The model under review builds one solid part; all positions refer to its coordinate system, in mm. A direction names the side the tool comes from. Round coordinates to 2 decimals unless told otherwise and drop trailing zeros. Loops run counter-clockwise (first coordinate to the right, second up) from the corner with the lowest first, then second, coordinate; pieces in that order, holes last. Notation, with made-up numbers: M 85,-11 L 143,-11 A8 ccw 143,1 Z; hole C 84.25,85 d7. An arc over 180 degrees is marked long. One line per question, with ' | ' between items.
from build123d import *

# Parameters (mm, degrees)
BOSS_EXTRUDE1_DEPTH = 9.525
BOSS_EXTRUDE2_START = -3.175
BOSS_EXTRUDE2_DEPTH = 3.175
FILLET1_R           = 9.525
SKETCH2_R           = 4.7625
SKETCH2_R_2         = 3.175
CUT_EXTRUDE1_DEPTH  = 71.245753875
SKETCH2_4_R         = 3.175
CUT_EXTRUDE2_DEPTH  = 71.245753961
CUT_EXTRUDE4_START  = -12.7
SKETCH2_6_R         = 4.7625
SKETCH2_6_R_2       = 3.175
CUT_EXTRUDE4_DEPTH  = 58.545753961


with BuildPart() as part:
    # Sketch1 → Boss-Extrude1 (new body)
    with BuildSketch(Plane.ZY.offset(50.8)):
        with BuildLine():
            ThreePointArc((12.636340451, 186.18), (-12.7, 187.45), (12.636340451, 188.72))
            Line((12.636340451, 188.72), (26.9875, 188.72))
            Line((26.9875, 188.72), (26.9875, 193.8))
            Line((26.9875, 193.8), (16.267034341, 193.8))
            ThreePointArc((16.267034341, 193.8), (-17.4625, 187.45), (16.267034341, 181.1))
            Line((16.267034341, 181.1), (26.9875, 181.1))
            Line((26.9875, 181.1), (26.9875, 186.18))
            Line((26.9875, 186.18), (12.636340451, 186.18))
        make_face()
    extrude(amount=BOSS_EXTRUDE1_DEPTH)

    # Sketch1<4> → Boss-Extrude2 (add)
    with BuildSketch(Plane.ZY.offset(50.8).offset(BOSS_EXTRUDE2_START)):
        with BuildLine():
            Line((17.416256953, 186.18), (14.256444382, 186.18))
            ThreePointArc((14.256444382, 186.18), (-14.3129, 187.45), (14.256444382, 188.72))
            Line((14.256444382, 188.72), (17.416256953, 188.72))
            ThreePointArc((17.416256953, 188.72), (17.032105803, 191.303086834), (16.267034341, 193.8))
            ThreePointArc((16.267034341, 193.8), (-17.4625, 187.45), (16.267034341, 181.1))
            ThreePointArc((16.267034341, 181.1), (17.032105803, 183.596913166), (17.416256953, 186.18))
        make_face()
        with BuildLine():
            ThreePointArc((16.267034341, 193.8), (17.032105803, 191.303086834), (17.416256953, 188.72))
            Line((17.416256953, 188.72), (26.9875, 188.72))
            Line((26.9875, 188.72), (26.9875, 193.8))
            Line((26.9875, 193.8), (16.267034341, 193.8))
        make_face()
        with BuildLine():
            Line((26.9875, 186.18), (17.416256953, 186.18))
            ThreePointArc((17.416256953, 186.18), (17.032105803, 183.596913166), (16.267034341, 181.1))
            Line((16.267034341, 181.1), (26.9875, 181.1))
            Line((26.9875, 181.1), (26.9875, 186.18))
        make_face()
    extrude(amount=BOSS_EXTRUDE2_DEPTH)

    # Fillet1
    fillet1_edges = [part.edges().sort_by_distance(p)[0] for p in [
        (-53.975, 181.1, 16.267034341),
        (-53.975, 193.8, 16.267034341),
    ]]
    fillet(fillet1_edges, radius=FILLET1_R)

    # Sketch2 → Cut-Extrude1 (cut, through all)
    # profile 1 of 2: a face of its own
    with BuildSketch(Plane(origin=(0, 193.8, 0), x_dir=(1, 0, 0), z_dir=(0, 1, 0))):
        with Locations((-53.975, -21.62726717)):
            Circle(SKETCH2_R)
        with Locations((-53.975, -21.62726717)):
            Circle(SKETCH2_R_2, mode=Mode.SUBTRACT)
    # profile 2 of 2: a face of its own
    with BuildSketch(Plane(origin=(0, 193.8, 0), x_dir=(1, 0, 0), z_dir=(0, 1, 0))):
        with Locations((-53.975, -21.62726717)):
            Circle(SKETCH2_R_2)
    extrude(amount=CUT_EXTRUDE1_DEPTH, mode=Mode.SUBTRACT)

    # Sketch2<4> → Cut-Extrude2 (cut, through all)
    with BuildSketch(Plane(origin=(0, 193.8, 0), x_dir=(1, 0, 0), z_dir=(0, 1, 0))):
        with Locations(Location((-53.975, -21.62726717, 0), (0, 0, 270))):
            Circle(SKETCH2_4_R)
    extrude(amount=-CUT_EXTRUDE2_DEPTH, mode=Mode.SUBTRACT)

    # Sketch2<6> → Cut-Extrude4 (cut, through all)
    # profile 1 of 3: a face of its own
    with BuildSketch(Plane(origin=(0, 193.8, 0), x_dir=(1, 0, 0), z_dir=(0, 1, 0)).offset(CUT_EXTRUDE4_START)):
        Polygon((-60.325, -21.513289799), (-60.325, -21.741244542), (-57.296072999, -26.9875), (-50.653927001, -26.9875), (-47.625, -21.741244542), (-47.625, -21.513289799), (-50.653927001, -16.267034341), (-57.296072999, -16.267034341), align=None)
        with Locations((-53.975, -21.62726717)):
            Circle(SKETCH2_6_R, mode=Mode.SUBTRACT)
    # profile 2 of 3: a face of its own
    with BuildSketch(Plane(origin=(0, 193.8, 0), x_dir=(1, 0, 0), z_dir=(0, 1, 0)).offset(CUT_EXTRUDE4_START)):
        with Locations((-53.975, -21.62726717)):
            Circle(SKETCH2_6_R)
        with Locations(Location((-53.975, -21.62726717, 0), (0, 0, 270))):
            Circle(SKETCH2_6_R_2, mode=Mode.SUBTRACT)
    # profile 3 of 3: a face of its own
    with BuildSketch(Plane(origin=(0, 193.8, 0), x_dir=(1, 0, 0), z_dir=(0, 1, 0)).offset(CUT_EXTRUDE4_START)):
        with Locations(Location((-53.975, -21.62726717, 0), (0, 0, 270))):
            Circle(SKETCH2_6_R_2)
    extrude(amount=-CUT_EXTRUDE4_DEPTH, mode=Mode.SUBTRACT)


solid = part.part
1) Machinability: for faces 1 (the cylindrical face through (-49.2, 186.8, -14.3)), 2 (the cylindrical face through (-54.064, 195.369, 16.587)), 3 (the flat face through (-54, 181.1, 25)), 4 (the flat face through (-54, 188.72, 18)), 5 (the flat face through (-54, 193.8, 25)), which of the approach directions +Z, -Z, +X, -X, +Y, -Y give a long, thin tool a straight path to every point of the face, cutting with its end or side? Answer none if there is none.
Output values:
face 1: +X | face 2: +Z, +X, -X, +Y | face 3: +Z, -Y | face 4: +Z, +X, -X | face 5: +Z, +Y
2) Mouldability with a two-part tool opening along Z and no side actions: class faces 6 (the cylindrical face through (-57.074, 183.676, 20.939)), 7 (the cylindrical face through (-53.89, 188.06, -17.45)), 8 (the flat face through (-60.325, 189, 13)), 9 (the cylindrical face through (-55.5, 186.91, -12.69)) as +Z half, -Z half, draft (parallel to the pull), parting line (faces both ways), or undercut.
Output values:
face 6: undercut | face 7: parting line | face 8: draft | face 9: undercut
3) Add section D-D on y = 180. State the section outline as (x, z) points (3 decimals), then the cut area to 3 significant figures.
Output values:
outline: M -60.325,-15.794 L -47.625,-15.794 L -47.625,-12.221 L -50.8,-12.221 L -50.8,-10.285 L -60.325,-10.285 Z; M -60.325,10.285 L -50.8,10.285 L -50.8,12.221 L -47.625,12.221 L -47.625,17.381 L -50.011,17.381 L -50.654,16.267 L -57.296,16.267 L -57.939,17.381 L -60.325,17.381 Z | area: 140 mm²
4) For line 1 (Z direction, x = -52.75, y = 184); line 2 (Y direction, x = -56, z = 0); line 3 (Z direction, x = -56.25, y = 187.45), list the stretches that pass through material, from the lowest coordinate up.
Output values:
line 1: z = -17.12 to -12.22, 12.22 to 18.7, 24.56 to 26.99 | line 2: y = 169.99 to 174.75, 200.15 to 204.91 | line 3: z = -17.46 to -12.7
5) Add section A-A on y = 184.5. State how many separate pieces and enclosed holes the cut face has, then the cut area to 3 significant figures.
Output values:
separate pieces: 2 | enclosed holes: 1 | area: 205 mm²
6) Insertion check: P1, Ø1.5, axis at x = -55, z = 18, coming from the -Y side; P2, Ø4, axis at y = 174.5, z = 16, coming from the +X side; P3, Ø2, axis at x = -51, y = 173.5, coming from the +Z side; P4, Ø1, axis at x = -54.5, y = 192.5, coming from the -Z side. Each pin has a flat end and moves straight along its axis. Give the tip position at first contact, or say it passes through.
Output values:
P1: stops at y = 181.1 | P2: passes through | P3: stops at z = 11.71 | P4: stops at z = -16.86
